Could you check a few things on this model? Use its own coordinates, in mm. Give positions to 0.01 mm unless a question says otherwise; leave off trailing zeros. Loops run counter-clockwise (first coordinate to the right, second up) from the corner with the lowest first, then second, coordinate; pieces in that order, holes last. Notation, with made-up numbers: (-16, -30) -> (31, -30) arc R7 ccw to (31, -23) -> close; hole circle Ø2 at (-16.5, 72). An arc over 180 degrees is marked (long way). Put each result on its own line as item: value.
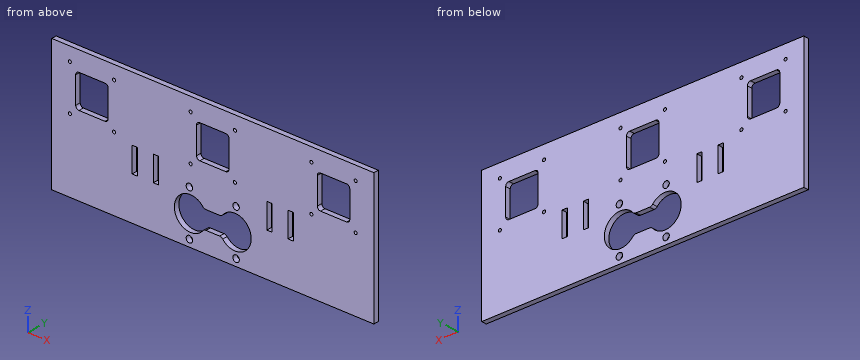
```python
from build123d import *

# Parameters (mm, degrees)
SKETCH1_W           = 200
SKETCH1_H           = 80
BOSS_EXTRUDE1_DEPTH = 3.175
SKETCH3_W           = 20.17
SKETCH3_H           = 20.17
CUT_EXTRUDE2_DEPTH  = 108.750084107
SKETCH5_R           = 2
CUT_EXTRUDE3_DEPTH  = 108.750084107
SKETCH6_R           = 0.95
CUT_EXTRUDE4_DEPTH  = 108.750084107
CUT_EXTRUDE5_DEPTH  = 108.750084107
FILLET1_R           = 2


with BuildPart() as part:
    # Sketch1 → Boss-Extrude1 (new body)
    with BuildSketch(Plane(origin=(0, 0, 0), x_dir=(1, 0, 0), z_dir=(0, 1, 0))):
        Rectangle(SKETCH1_W, SKETCH1_H)
    extrude(amount=BOSS_EXTRUDE1_DEPTH)

    # Sketch3 → Cut-Extrude2 (cut, through all)
    with BuildSketch(Plane(origin=(0, 3.175, 0), x_dir=(1, 0, 0), z_dir=(0, 1, 0))):
        with Locations((75, -18)):
            Rectangle(SKETCH3_W, SKETCH3_H)
        with Locations((-75, -18)):
            Rectangle(SKETCH3_W, SKETCH3_H)
        with Locations((0, -18)):
            Rectangle(SKETCH3_W, SKETCH3_H)
        with BuildLine():
            Line((4.245313644, 27.5), (-4.245313644, 27.5))
            ThreePointArc((-4.245313644, 27.5), (-5.305973816, 27.736153715), (-6.166250915, 28.4))
            ThreePointArc((-6.166250915, 28.4), (-23.85, 22), (-6.166250915, 15.6))
            ThreePointArc((-6.166250915, 15.6), (-5.305973816, 16.263846285), (-4.245313644, 16.5))
            Line((-4.245313644, 16.5), (4.245313644, 16.5))
            ThreePointArc((4.245313644, 16.5), (5.305973816, 16.263846285), (6.166250915, 15.6))
            ThreePointArc((6.166250915, 15.6), (23.85, 22), (6.166250915, 28.4))
            ThreePointArc((6.166250915, 28.4), (5.305973816, 27.736153715), (4.245313644, 27.5))
        make_face()
    extrude(amount=-CUT_EXTRUDE2_DEPTH, mode=Mode.SUBTRACT)

    # Sketch5 → Cut-Extrude3 (cut, through all)
    with BuildSketch(Plane.XZ):
        with Locations(Location((14.5, -8.2, 0), (0, 0, 270))):
            Circle(SKETCH5_R)
        with Locations(Location((-14.5, -8.2, 0), (0, 0, 270))):
            Circle(SKETCH5_R)
        with Locations(Location((14.5, -35.8, 0), (0, 0, 270))):
            Circle(SKETCH5_R)
        with Locations(Location((-14.5, -35.8, 0), (0, 0, 270))):
            Circle(SKETCH5_R)
    extrude(amount=-CUT_EXTRUDE3_DEPTH, mode=Mode.SUBTRACT)

    # Sketch6 → Cut-Extrude4 (cut, through all)
    with BuildSketch(Plane.XZ):
        with Locations(Location((-61.25, 4.25, 0), (0, 0, 270))):
            Circle(SKETCH6_R)
        with Locations(Location((13.75, 4.25, 0), (0, 0, 270))):
            Circle(SKETCH6_R)
        with Locations(Location((-88.75, 4.25, 0), (0, 0, 270))):
            Circle(SKETCH6_R)
        with Locations(Location((-61.25, 31.75, 0), (0, 0, 270))):
            Circle(SKETCH6_R)
        with Locations(Location((-13.75, 4.25, 0), (0, 0, 270))):
            Circle(SKETCH6_R)
        with Locations(Location((-13.75, 31.75, 0), (0, 0, 270))):
            Circle(SKETCH6_R)
        with Locations(Location((13.75, 31.75, 0), (0, 0, 270))):
            Circle(SKETCH6_R)
        with Locations(Location((88.75, 31.75, 0), (0, 0, 270))):
            Circle(SKETCH6_R)
        with Locations(Location((61.25, 31.75, 0), (0, 0, 270))):
            Circle(SKETCH6_R)
        with Locations(Location((61.25, 4.25, 0), (0, 0, 270))):
            Circle(SKETCH6_R)
        with Locations(Location((88.75, 4.25, 0), (0, 0, 270))):
            Circle(SKETCH6_R)
        with Locations(Location((-88.75, 31.75, 0), (0, 0, 270))):
            Circle(SKETCH6_R)
    extrude(amount=-CUT_EXTRUDE4_DEPTH, mode=Mode.SUBTRACT)

    # Sketch7 → Cut-Extrude5 (cut, through all)
    with BuildSketch(Plane(origin=(0, 3.175, 0), x_dir=(1, 0, 0), z_dir=(0, 1, 0))):
        Polygon((-50.1, 13.925), (-50.1, 12.825), (-50.1, -0.175), (-50.1, -1.275), (-46.725, -1.275), (-46.725, -0.175), (-46.725, 12.825), (-46.725, 13.925), align=None)
        Polygon((-36.925, -0.175), (-36.925, -1.275), (-33.55, -1.275), (-33.55, -0.175), (-33.55, 12.825), (-33.55, 13.925), (-36.925, 13.925), (-36.925, 12.825), align=None)
        Polygon((33.55, 13.925), (33.55, 12.825), (33.55, -0.175), (33.55, -1.275), (36.925, -1.275), (36.925, -0.175), (36.925, 12.825), (36.925, 13.925), align=None)
        Polygon((46.725, -0.175), (46.725, -1.275), (50.1, -1.275), (50.1, -0.175), (50.1, 12.825), (50.1, 13.925), (46.725, 13.925), (46.725, 12.825), align=None)
    extrude(amount=-CUT_EXTRUDE5_DEPTH, mode=Mode.SUBTRACT)

    # Fillet1
    fillet1_edges = [part.edges().sort_by_distance(p)[0] for p in [
        (85.085, 1.5875, 7.915),
        (85.085, 1.5875, 28.085),
        (64.915, 1.5875, 28.085),
        (64.915, 1.5875, 7.915),
        (-64.915, 1.5875, 7.915),
        (-64.915, 1.5875, 28.085),
        (-85.085, 1.5875, 28.085),
        (-85.085, 1.5875, 7.915),
        (10.085, 1.5875, 7.915),
        (10.085, 1.5875, 28.085),
        (-10.085, 1.5875, 28.085),
        (-10.085, 1.5875, 7.915),
    ]]
    fillet(fillet1_edges, radius=FILLET1_R)


solid = part.part
```
1. I need wall thicknesses on line 1 (X direction, y = 1.2, z = 24.5) (3 decimals); line 2 (X direction, y = 0.7, z = -1.5) (3 decimals); line 3 (X direction, y = 0.85, z = -36). Which ranges of each line are inside material? Lowest first, please.
Recorded:
line 1: x = -100 to -85.085, -64.915 to -10.085, 10.085 to 64.915, 85.085 to 100
line 2: x = -100 to -50.1, -46.725 to -36.925, -33.55 to 33.55, 36.925 to 46.725, 50.1 to 100
line 3: x = -100 to -16.49, -12.51 to 12.51, 16.49 to 100
2. If we section it at B-B (z = -22): List the corners of the cut face in (x, y) for me (3 decimals).
Recorded:
outline: (-100, 0) -> (-23.85, 0) -> (-23.85, 3.175) -> (-100, 3.175) -> close; (23.85, 0) -> (100, 0) -> (100, 3.175) -> (23.85, 3.175) -> close
3. If we section it at A-A (z = 21.5): List the corners of the cut face in (x, y) for me (3 decimals), then the cut area to 3 significant figures.
Recorded:
outline: (-100, 0) -> (-85.085, 0) -> (-85.085, 3.175) -> (-100, 3.175) -> close; (-64.915, 0) -> (-10.085, 0) -> (-10.085, 3.175) -> (-64.915, 3.175) -> close; (10.085, 0) -> (64.915, 0) -> (64.915, 3.175) -> (10.085, 3.175) -> close; (85.085, 0) -> (100, 0) -> (100, 3.175) -> (85.085, 3.175) -> close
area: 443 mm^2
4. If we section it at C-C (x = 19): List the corners of the cut face in (y, z) for me (3 decimals), then the cut area to 3 significant figures.
Recorded:
outline: (0, -40) -> (3.175, -40) -> (3.175, -30.572) -> (0, -30.572) -> close; (0, -13.428) -> (3.175, -13.428) -> (3.175, 40) -> (0, 40) -> close
area: 200 mm^2
5. If we section it at D-D (y = 0.7): Count the separate pieces of the cut face and the enclosed holes in it, then the cut area to 3 significant figures.
Recorded:
separate pieces: 1
enclosed holes: 24
area: 13,800 mm^2
6. I'm going to push a flat-ended pin straight in: pin 1 (2.5 mm diameter, centred on x = 88.75, z = 31.75, fed in from +Y) (3 decimals). Where does the tip first touch, or does it pass through?
Recorded:
pin 1: stops at y = 3.175
